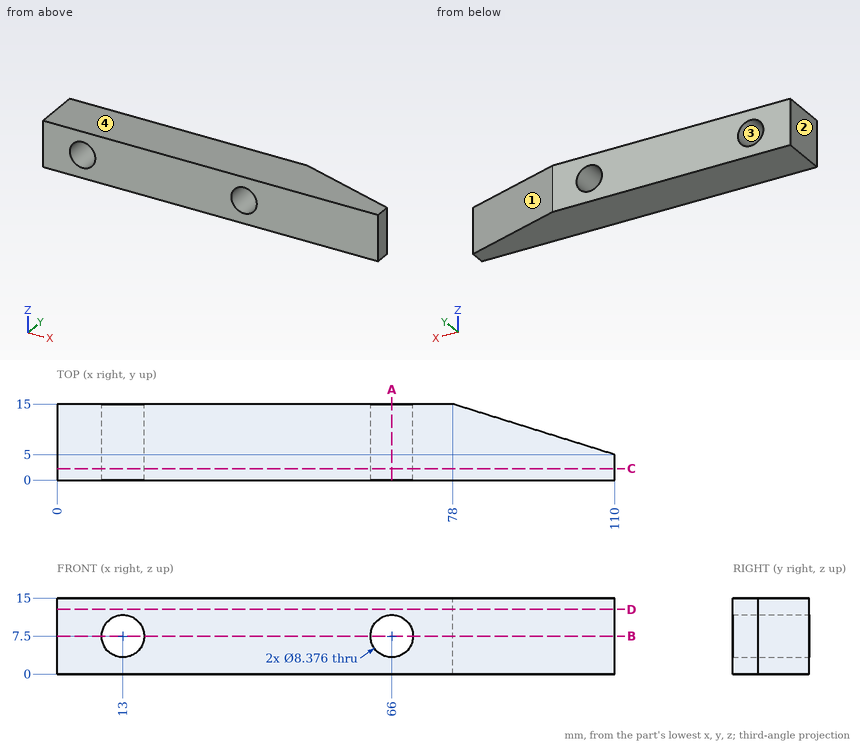
Geometry: see drawing. Coordinates: mm, zero at the bounding-box minimum. Give positions to 0.01 mm unless a question says otherwise; leave off trailing zeros. Order: outer loops, then holes, each group sorted by start corner. A loop starts at its lowest first (then second) coordinate and runs counter-clockwise, first axis right, second up. Notation, with made-up numbers: (86.25, -22.5) -> (140.25, -22.5) arc R23 ccw to (140.25, -0.5) -> close; hole circle Ø11 at (-23.5, 69.5). An arc over 180 degrees is marked (long way). Write each question's results on one line, items separated by ' | '. Start each with the question number.
1) Draft query along X for the marked faces 1, 2, 3 and 4. Return one class per face: pulls with the +X half, pulls with the -X half, needs draft (parallel to the pull), parting line crosses it, or undercut.
2) Section B-B (z = 7.5). Return loops of the section in (x, y), then the cut area to 3 significant figures.
3) Section D-D (z = 12.75). Return loops of the section in (x, y), then the cut area to 3 significant figures.
4) Section A-A (x = 66). Return loops of the section in (y, z).
5) Section C-C (y = 2.25). Return loops of the section in (x, z), then the cut area to 3 significant figures.
6) Line query: line 1 (X direction, y = 3, z = 7.5); line 2 (Z direction, x = 13, y = 6.25); line 3 (X direction, y = 4.25, z = 5.5). Output: solid intervals per line, ascending. Write a range as from..to.
Calculated:
1) face 1: pulls with the +X half | face 2: pulls with the -X half | face 3: undercut | face 4: needs draft
2) outline: (0, 0) -> (8.81, 0) -> (8.81, 15) -> (0, 15) -> close; (17.19, 0) -> (61.81, 0) -> (61.81, 15) -> (17.19, 15) -> close; (70.19, 0) -> (110, 0) -> (110, 5) -> (78, 15) -> (70.19, 15) -> close | area: 1,240 mm2
3) outline: (0, 0) -> (110, 0) -> (110, 5) -> (78, 15) -> (0, 15) -> close | area: 1,490 mm2
4) outline: (0, 0) -> (15, 0) -> (15, 3.31) -> (0, 3.31) -> close; (0, 11.69) -> (15, 11.69) -> (15, 15) -> (0, 15) -> close
5) outline: (0, 0) -> (110, 0) -> (110, 15) -> (0, 15) -> close; hole circle Ø8.38 at (13, 7.5); hole circle Ø8.38 at (66, 7.5) | area: 1,540 mm2
6) line 1: 0..8.81, 17.19..61.81, 70.19..110 | line 2: 0..3.31, 11.69..15 | line 3: 0..9.32, 16.68..62.32, 69.68..110
